```python
from build123d import *

# Parameters (mm, degrees)
F0_W     = 13
F0_H     = 13
F1_DEPTH = 40
F3_DEPTH = 6.5
F5_D     = 3.3
F6_D     = 4.2


with BuildPart() as f1:
    # F0 (on Front) → F1 (new body, symmetric)
    with BuildSketch(Plane.XZ):
        Rectangle(F0_W, F0_H)
    extrude(amount=F1_DEPTH, both=True)

    # F2 (on Right) → F3 (cut, symmetric)
    with BuildSketch(Plane.YZ):
        with BuildLine():
            ThreePointArc((0, -3.3166247904), (11, 0), (0, 3.3166247904))
            ThreePointArc((0, 3.3166247904), (-11, 0), (0, -3.3166247904))
        make_face()
    extrude(amount=F3_DEPTH, both=True, mode=Mode.SUBTRACT)

    # F5 (through all)
    with Locations(Plane.XY.offset(6.5)):
        with Locations((0, -35), (0, -20)):
            Hole(F5_D / 2)

    # F6 (through all)
    with Locations(Plane.XY.offset(6.5)):
        with Locations((0, 20), (0, 35)):
            Hole(F6_D / 2)


solid = f1.part
```
Work out the finished part from the listing and answer in its coordinate system (mm). Coordinates: 2 decimals unless noted, no trailing zeros. Loops run counter-clockwise (first coordinate to the right, second up) from the corner with the lowest first, then second, coordinate; pieces in that order, holes last. Notation, with made-up numbers: (-14.5, 55.25) - (11.5, 55.25) arc R7 cw to (11.5, 60.25) - close; hole circle Ø6 at (39, 9). An arc over 180 degrees is marked (long way). Use a Markdown table: item, result.
Item 1: Given pin 1 Ø5 at (x, y) = (0, 35) entering from -Z, flat-ended and moving along its own axis, determine where the tip first touches the part or whether it passes through.
Evaluation:
| item | result |
|---|---|
| pin 1 | stops at z = -6.5 |
Item 2: Consider probe 1 along Y at (x, z) = (0, -2.5); probe 2 along Y at (x, z) = (1.5, 0); probe 3 along Z at (x, y) = (-1, 5). Determine where each line is inside the solid, lowest interval first. Write a range as from..to.
Evaluation:
| item | result |
|---|---|
| probe 1 | y = -40..-36.65, -33.35..-21.65, -18.35..-10.45, 10.45..17.9, 22.1..32.9, 37.1..40 |
| probe 2 | y = -40..-35.69, -34.31..-20.69, -19.31..-11, 11..18.53, 21.47..33.53, 36.47..40 |
| probe 3 | z = -6.5..-6, 6..6.5 |
Item 3: Find section A-A, the plane y = 20. Determine the outline of the cut face in (x, z), and give its area (3 significant figures).
Evaluation:
| item | result |
|---|---|
| outline | (-6.5, -6.5) - (-2.1, -6.5) - (-2.1, 6.5) - (-6.5, 6.5) - close; (2.1, -6.5) - (6.5, -6.5) - (6.5, 6.5) - (2.1, 6.5) - close |
| area | 114 mm2 |
Item 4: Find section D-D, the plane x = 5. Determine the outline of the cut face in (y, z).
Evaluation:
| item | result |
|---|---|
| outline | (-40, -6.5) - (40, -6.5) - (40, 6.5) - (-40, 6.5) - close; hole (0, -3.32) arc R6 ccw (long way) to (0, 3.32) arc R6 ccw (long way) to start |
Item 5: Find section B-B, the plane z = 1.75. Determine the outline of the cut face in (x, y).
Evaluation:
| item | result |
|---|---|
| outline | (-6.5, -40) - (6.5, -40) - (6.5, -10.74) - (-6.5, -10.74) - close; (-6.5, 10.74) - (6.5, 10.74) - (6.5, 40) - (-6.5, 40) - close; hole circle Ø4.2 at (0, 20); hole circle Ø4.2 at (0, 35); hole circle Ø3.3 at (0, -35); hole circle Ø3.3 at (0, -20) |
Item 6: The mould has two halves that part along Z. Classify faces 1 (the flat face through (0, -1, 6.5)), 2 (the cylindrical face through (-0.89, -33.61, -0.09)), 3 (the cylindrical face through (0, 11, 0)): +Z half, -Z half, draft (parallel to the pull), parting line (faces both ways), or undercut.
Evaluation:
| item | result |
|---|---|
| face 1 | +Z half |
| face 2 | draft |
| face 3 | undercut |
Item 7: Find section C-C, the plane z = -4. Determine the outline of the cut face in (x, y), and give its area (3 significant figures).
Evaluation:
| item | result |
|---|---|
| outline | (-6.5, -40) - (6.5, -40) - (6.5, -9.47) - (-6.5, -9.47) - close; (-6.5, -0.53) - (6.5, -0.53) - (6.5, 0.53) - (-6.5, 0.53) - close; (-6.5, 9.47) - (6.5, 9.47) - (6.5, 40) - (-6.5, 40) - close; hole circle Ø4.2 at (0, 20); hole circle Ø4.2 at (0, 35); hole circle Ø3.3 at (0, -35); hole circle Ø3.3 at (0, -20) |
| area | 763 mm2 |
